```python
from build123d import *

# Parameters (mm, degrees)
SKETCH1_W           = 86
SKETCH1_H           = 86
BOSS_EXTRUDE1_DEPTH = 101.6
SKETCH2_R           = 36.5
BOSS_EXTRUDE2_DEPTH = 1.6
SKETCH3_R           = 7
BOSS_EXTRUDE3_DEPTH = 37
SKETCH5_R           = 3.25
CUT_EXTRUDE1_DEPTH  = 102.6
SKETCH4_W           = 16.3
SKETCH4_H           = 16.3
CUT_EXTRUDE2_DEPTH  = 91.6
FILLET1_R           = 6.35


with BuildPart() as part:
    # Sketch1 → Boss-Extrude1 (new body)
    with BuildSketch(Plane.XY):
        Rectangle(SKETCH1_W, SKETCH1_H)
    extrude(amount=-BOSS_EXTRUDE1_DEPTH)

    # Sketch2 → Boss-Extrude2 (add)
    with BuildSketch(Plane.XY):
        Circle(SKETCH2_R)
    extrude(amount=BOSS_EXTRUDE2_DEPTH)

    # Sketch3 → Boss-Extrude3 (add)
    with BuildSketch(Plane.XY.offset(1.6)):
        Circle(SKETCH3_R)
    extrude(amount=BOSS_EXTRUDE3_DEPTH)

    # Sketch5 → Cut-Extrude1 (cut, through all)
    with BuildSketch(Plane.XY):
        with Locations((-34.85, 34.85)):
            Circle(SKETCH5_R)
        with Locations((34.85, 34.85)):
            Circle(SKETCH5_R)
        with Locations((34.85, -34.85)):
            Circle(SKETCH5_R)
        with Locations((-34.85, -34.85)):
            Circle(SKETCH5_R)
    extrude(amount=-CUT_EXTRUDE1_DEPTH, mode=Mode.SUBTRACT)

    # Sketch4 → Cut-Extrude2 (cut)
    with BuildSketch(Plane(origin=(0, 0, -101.6), x_dir=(-1, 0, 0), z_dir=(0, 0, -1))):
        with Locations((-34.85, 34.85)):
            Rectangle(SKETCH4_W, SKETCH4_H)
        with Locations((-34.85, -34.85)):
            Rectangle(SKETCH4_W, SKETCH4_H)
        with Locations((34.85, -34.85)):
            Rectangle(SKETCH4_W, SKETCH4_H)
        with Locations((34.85, 34.85)):
            Rectangle(SKETCH4_W, SKETCH4_H)
    extrude(amount=-CUT_EXTRUDE2_DEPTH, mode=Mode.SUBTRACT)

    # Fillet1
    fillet1_edges = [part.edges().sort_by_distance(p)[0] for p in [
        (43, 43, -5),
        (-43, 43, -5),
        (-43, -43, -5),
        (43, -43, -5),
        (-26.7, 26.7, -55.8),
        (-26.7, -26.7, -55.8),
        (26.7, -26.7, -55.8),
        (26.7, 26.7, -55.8),
    ]]
    fillet(fillet1_edges, radius=FILLET1_R)


solid = part.part
```
Verification items for the finished model (mm, model axes). A direction names the side the tool comes from. Coordinates: 2 decimals unless noted, no trailing zeros. Loops run counter-clockwise (first coordinate to the right, second up) from the corner with the lowest first, then second, coordinate; pieces in that order, holes last. Notation, with made-up numbers: (-27, 86.25) - (21, 86.25) arc R23 ccw to (21, 120.25) - close; hole circle Ø11 at (53.5, 81). An arc over 180 degrees is marked (long way). Answer as a JSON object with one key per item and string values.
(1) Cross-section at B-B, the plane x = -34.85. Record the boundary of the cut face in (y, z), then the cut area to 3 significant figures.
Response:
{"outline": "(-43, -10) - (-38.1, -10) - (-38.1, 0) - (-43, 0) - close; (-31.6, -10) - (-26.7, -10) - (-26.7, -101.6) - (26.7, -101.6) - (26.7, -10) - (31.6, -10) - (31.6, 0) - (10.85, 0) - (10.85, 1.6) - (-10.85, 1.6) - (-10.85, 0) - (-31.6, 0) - close; (38.1, -10) - (43, -10) - (43, 0) - (38.1, 0) - close", "area": "5,660 mm²"}
(2) Cross-section at D-D, the plane z = -88. Record the boundary of the cut face in (x, y).
Response:
{"outline": "(-43, -26.7) - (-33.05, -26.7) arc R6.35 cw to (-26.7, -33.05) - (-26.7, -43) - (26.7, -43) - (26.7, -33.05) arc R6.35 cw to (33.05, -26.7) - (43, -26.7) - (43, 26.7) - (33.05, 26.7) arc R6.35 cw to (26.7, 33.05) - (26.7, 43) - (-26.7, 43) - (-26.7, 33.05) arc R6.35 cw to (-33.05, 26.7) - (-43, 26.7) - close"}
(3) Cross-section at A-A, the plane y = 0. Record the boundary of the cut face in (x, z).
Response:
{"outline": "(-43, -101.6) - (43, -101.6) - (43, 0) - (36.5, 0) - (36.5, 1.6) - (7, 1.6) - (7, 38.6) - (-7, 38.6) - (-7, 1.6) - (-36.5, 1.6) - (-36.5, 0) - (-43, 0) - close"}
(4) Scan lines: line 1 along Y through (x, z) = (-34.85, -5.5); line 2 along X through (y, z) = (-34, -7). Record each from-to range of solid material in increasing order.
Response:
{"line 1": "y = -43 to -38.1, -31.6 to 31.6, 38.1 to 43", "line 2": "x = -43 to -37.99, -31.71 to 31.71, 37.99 to 43"}
(5) Access from +Z, -Z, +X, -X, +Y, -Y to the whole of each face (thin tool, end or side, straight path). Record for faces 1 (the flat face through (38, -26.7, -56)), 2 (the flat face through (-26.7, 38, -56)), 3 (the flat face through (35, 39, -10)), 4 (the flat face through (38, 1, 0)), 5 (the cylindrical face through (-28.61, -28.51, -55.16)).
Response:
{"face 1": "-Z, +X, -Y", "face 2": "-Z, -X, +Y", "face 3": "-Z, +X, +Y", "face 4": "+Z", "face 5": "-Z, -X, -Y"}
(6) Go/stop test with flat-tipped pins: pin 1 Ø2 at (x, y) = (-22.5, 11) entering from +Z; pin 2 Ø11 at (y, z) = (-40, -33.5) entering from +X; pin 3 Ø5 at (x, y) = (38.5, 36) entering from -Z. Record where each tip stops, or that it passes through.
Response:
{"pin 1": "stops at z = 1.6", "pin 2": "stops at x = 26.7", "pin 3": "stops at z = -10"}
